Read the model definition and answer for the solid it produces. Units are mm, in the model's axes. A direction names the side the tool comes from. Give positions to 0.01 mm unless a question says otherwise; leave off trailing zeros. Loops run counter-clockwise (first coordinate to the right, second up) from the corner with the lowest first, then second, coordinate; pieces in that order, holes last. Notation, with made-up numbers: (-11, 11.5) - (-3, 11.5) arc R30 cw to (-3, 37.5) - close; hole circle Ø10 at (39.25, 47.5). An arc over 180 degrees is marked (long way). Use a Markdown table: item, result. Add a question column.
Item 1: Which of the six approach directions +Z, -Z, +X, -X, +Y, -Y give full straight-line access (tool end or side, diameter ignored) to faces 1 (the face through (4.8, 4.2, 10.3)), 2 (the face through (-7, 0, 6))?
Item 2: For a pull along Z with two mould halves and no side action, classify faces 3 (the face through (9.23, 6.08, -12.9)), 4 (the face through (2, 6, -19.759)), 5 (the face through (-17.521, 6, 7)) as +Z half, -Z half, draft (parallel to the pull), parting line (faces both ways), or undercut.
Item 3: A cutting plane is placed at B-B (y = 10). Determine the outline of the cut face in (x, z).
Item 4: A cutting plane is placed at D-D (z = 13). Determine the outline of the cut face in (x, y), plus the area to 3 significant figures.
Item 5: A cutting plane is placed at A-A (z = 24.5). Determine the outline of the cut face in (x, y).
Item 6: A cutting plane is placed at C-C (x = -6.5). Determine the outline of the cut face in (y, z), plus the area to 3 significant figures.
Item 7: Consider probe 1 along X at (y, z) = (3.5, -12.5); probe 2 along X at (y, z) = (9, 24); probe 3 along Z at (x, y) = (-9.5, 1.75). Determine where each line is inside the solid, lowest interval first. Write a range as [from, to].
Item 8: Each of these flat-tipped pins is pushed along its axis until it touches: P1, Ø9.5, axis at x = 3, z = 5, coming from the -Y side; P2, Ø6, axis at x = -7.52, z = -12.76, coming from the +Y side. Where does it stop, or does it pass through?
from build123d import *

# Parameters (mm, degrees)
SKETCH1_W           = 40
SKETCH1_H           = 53
BOSS_EXTRUDE1_DEPTH = 12
SKETCH2_R           = 8
CUT_EXTRUDE1_DEPTH  = 3.5
SKETCH4_R           = 4.25
CUT_EXTRUDE2_DEPTH  = 1.5
CUT_EXTRUDE3_REACH  = 14
SKETCH5_R           = 3.25


with BuildPart() as part:
    # Sketch1 → Boss-Extrude1 (new body)
    with BuildSketch(Plane(origin=(0, 0, 0), x_dir=(1, 0, 0), z_dir=(0, 1, 0))):
        with Locations((2.478549399, -6.741379093)):
            Rectangle(SKETCH1_W, SKETCH1_H)
    extrude(amount=BOSS_EXTRUDE1_DEPTH)

    # Sketch2 → Cut-Extrude1 (cut)
    with BuildSketch(Plane.XZ):
        with Locations((2.478549399, 6.741379093)):
            Circle(SKETCH2_R)
    extrude(amount=-CUT_EXTRUDE1_DEPTH, mode=Mode.SUBTRACT)

    # Sketch4 → Cut-Extrude2 (cut)
    with BuildSketch(Plane.XZ.offset(-3.5)):
        with Locations((2.478549399, 6.741379093)):
            Circle(SKETCH4_R)
    extrude(amount=-CUT_EXTRUDE2_DEPTH, mode=Mode.SUBTRACT)

    # Sketch5 → Cut-Extrude3 (cut, up to next)
    with BuildSketch(Plane(origin=(0, 12, 0), x_dir=(1, 0, 0), z_dir=(0, 1, 0)), mode=Mode.PRIVATE) as cut_extrude3_sk1:
        with Locations((-7.521450601, -26.241379093)):
            Circle(SKETCH5_R)
    cut_extrude3_tool1 = extrude(cut_extrude3_sk1.sketch, amount=-CUT_EXTRUDE3_REACH, mode=Mode.PRIVATE) & part.part
    add(cut_extrude3_tool1.solids().sort_by_distance((-7.521451, 12, 26.241379))[0], mode=Mode.SUBTRACT)
    # Sketch5 → Cut-Extrude3 (cut, up to next)
    with BuildSketch(Plane(origin=(0, 12, 0), x_dir=(1, 0, 0), z_dir=(0, 1, 0)), mode=Mode.PRIVATE) as cut_extrude3_sk2:
        with Locations((12.478549399, -26.241379093)):
            Circle(SKETCH5_R)
    cut_extrude3_tool2 = extrude(cut_extrude3_sk2.sketch, amount=-CUT_EXTRUDE3_REACH, mode=Mode.PRIVATE) & part.part
    add(cut_extrude3_tool2.solids().sort_by_distance((12.478549, 12, 26.241379))[0], mode=Mode.SUBTRACT)
    # Sketch5 → Cut-Extrude3 (cut, up to next)
    with BuildSketch(Plane(origin=(0, 12, 0), x_dir=(1, 0, 0), z_dir=(0, 1, 0)), mode=Mode.PRIVATE) as cut_extrude3_sk3:
        with Locations((-7.521450601, 12.758620907)):
            Circle(SKETCH5_R)
    cut_extrude3_tool3 = extrude(cut_extrude3_sk3.sketch, amount=-CUT_EXTRUDE3_REACH, mode=Mode.PRIVATE) & part.part
    add(cut_extrude3_tool3.solids().sort_by_distance((-7.521451, 12, -12.758621))[0], mode=Mode.SUBTRACT)
    # Sketch5 → Cut-Extrude3 (cut, up to next)
    with BuildSketch(Plane(origin=(0, 12, 0), x_dir=(1, 0, 0), z_dir=(0, 1, 0)), mode=Mode.PRIVATE) as cut_extrude3_sk4:
        with Locations((12.478549399, 12.758620907)):
            Circle(SKETCH5_R)
    cut_extrude3_tool4 = extrude(cut_extrude3_sk4.sketch, amount=-CUT_EXTRUDE3_REACH, mode=Mode.PRIVATE) & part.part
    add(cut_extrude3_tool4.solids().sort_by_distance((12.478549, 12, -12.758621))[0], mode=Mode.SUBTRACT)


solid = part.part
Geometry says:
| question | item | result |
|---|---|---|
| 1 | face 1 | -Y |
| 1 | face 2 | +Z, -Z, +X, -X, -Y |
| 2 | face 3 | undercut |
| 2 | face 4 | -Z half |
| 2 | face 5 | draft |
| 3 | outline | (-17.52, -19.76) - (22.48, -19.76) - (22.48, 33.24) - (-17.52, 33.24) - close; hole circle Ø6.5 at (-7.52, -12.76); hole circle Ø6.5 at (-7.52, 26.24); hole circle Ø6.5 at (12.48, -12.76); hole circle Ø6.5 at (12.48, 26.24) |
| 4 | outline | (-17.52, 0) - (-2.5, 0) - (-2.5, 3.5) - (7.46, 3.5) - (7.46, 0) - (22.48, 0) - (22.48, 12) - (-17.52, 12) - close |
| 4 | area | 445 mm² |
| 5 | outline | (-17.52, 0) - (-10.27, 0) - (-10.27, 12) - (-17.52, 12) - close; (-4.78, 0) - (9.73, 0) - (9.73, 12) - (-4.78, 12) - close; (15.22, 0) - (22.48, 0) - (22.48, 12) - (15.22, 12) - close |
| 6 | outline | (0, -19.76) - (12, -19.76) - (12, -15.84) - (0, -15.84) - close; (0, -9.67) - (12, -9.67) - (12, 23.16) - (0, 23.16) - close; (0, 29.33) - (12, 29.33) - (12, 33.24) - (0, 33.24) - close |
| 6 | area | 488 mm² |
| 7 | probe 1 | [-17.52, -10.76], [-4.28, 9.24], [15.72, 22.48] |
| 7 | probe 2 | [-17.52, -9.87], [-5.17, 10.13], [14.83, 22.48] |
| 7 | probe 3 | [-19.76, -15.34], [-10.18, 23.66], [28.82, 33.24] |
| 8 | P1 | y = 3.5 |
| 8 | P2 | through |
